Geometry: final body of the model. Coordinates: model frame, mm. A direction names the side the tool comes from. Round coordinates to 2 decimals unless told otherwise and drop trailing zeros. Order: outer loops, then holes, each group sorted by start corner. A loop starts at its lowest first (then second) coordinate and runs counter-clockwise, first axis right, second up. Notation, with made-up numbers: (-37, 17) -> (-27, 17) arc R20 cw to (-27, 25) -> close; hole circle Ø1 at (49.5, -30). An arc over 180 degrees is marked (long way). Put each result on its own line as item: value.
```python
from build123d import *

# Parameters (mm, degrees)
F0_R     = 3.048
F1_DEPTH = 3.175
F2_R     = 3.175


with BuildPart() as f1:
    # F0 (on Front) → F1 (new body)
    with BuildSketch(Plane.XZ):
        with BuildLine():
            ThreePointArc((-63.5, 3.175), (-62.570064, 0.929936), (-60.325, 0))
            Line((-60.325, 0), (60.325, 0))
            ThreePointArc((60.325, 0), (62.570064, 0.929936), (63.5, 3.175))
            Line((63.5, 3.175), (63.5, 27.559))
            ThreePointArc((63.5, 27.559), (62.570064, 29.804064), (60.325, 30.734))
            Line((60.325, 30.734), (7.62, 30.734))
            Line((7.62, 30.734), (-11.43, 26.924))
            Line((-11.43, 26.924), (-60.325, 26.924))
            ThreePointArc((-60.325, 26.924), (-62.570064, 25.994064), (-63.5, 23.749))
            Line((-63.5, 23.749), (-63.5, 3.175))
        make_face()
        with Locations((-40.64, 7.62)):
            Circle(F0_R, mode=Mode.SUBTRACT)
        with Locations((0, 7.62)):
            Circle(F0_R, mode=Mode.SUBTRACT)
        with Locations((40.64, 7.62)):
            Circle(F0_R, mode=Mode.SUBTRACT)
        with Locations((-53.34, 16.51)):
            Circle(F0_R, mode=Mode.SUBTRACT)
        with Locations((-25.4, 19.05)):
            Circle(F0_R, mode=Mode.SUBTRACT)
        with Locations((0, 19.05)):
            Circle(F0_R, mode=Mode.SUBTRACT)
        with Locations((25.4, 19.05)):
            Circle(F0_R, mode=Mode.SUBTRACT)
        with Locations((53.34, 16.51)):
            Circle(F0_R, mode=Mode.SUBTRACT)
    extrude(amount=F1_DEPTH)

    # F2
    f2_edges = [f1.edges().sort_by_distance(p)[0] for p in [
        (-11.43, -1.5875, 26.924),
        (7.62, -1.5875, 30.734),
    ]]
    fillet(f2_edges, radius=F2_R)


solid = f1.part
```
1. Cut plane C-C on y = -0.55. State how many separate pieces and enclosed holes the cut face has, and give its area (3 significant figures).
Ans:
separate pieces: 1
enclosed holes: 8
area: 3,430 mm²
2. Contact query for flat-ended pins moving along their axis: P1, Ø1.5, axis at x = -10.5, y = -1, coming from the +Z side; P2, Ø1, axis at y = -2, z = 26.5, coming from the -X side. Output: stop coordinate, or through.
Ans:
P1: z = 27.26
P2: x = -62.56
3. Cut plane D-D on x = 0. Return loops of the section in (y, z) (3 decimals).
Ans:
outline: (-3.175, 0) -> (0, 0) -> (0, 4.572) -> (-3.175, 4.572) -> close; (-3.175, 10.668) -> (0, 10.668) -> (0, 16.002) -> (-3.175, 16.002) -> close; (-3.175, 22.098) -> (0, 22.098) -> (0, 29.21) -> (-3.175, 29.21) -> close
4. Material intervals for probe 1 along Z at (x, y) = (25.4, -1.3); probe 2 along Z at (x, y) = (-25.4, -2.1); probe 3 along X at (y, z) = (-1.3, 21), sorted ascending.
Ans:
probe 1: 0 to 16, 22.1 to 30.73
probe 2: 0 to 16, 22.1 to 26.92
probe 3: -63.5 to -27.74, -23.06 to -2.34, 2.34 to 23.06, 27.74 to 63.5
5. Cut plane B-B on z = 7.62. Return loops of the section in (x, y) (3 decimals), and give its area (3 significant figures).
Ans:
outline: (-63.5, -3.175) -> (-43.688, -3.175) -> (-43.688, 0) -> (-63.5, 0) -> close; (-37.592, -3.175) -> (-3.048, -3.175) -> (-3.048, 0) -> (-37.592, 0) -> close; (3.048, -3.175) -> (37.592, -3.175) -> (37.592, 0) -> (3.048, 0) -> close; (43.688, -3.175) -> (63.5, -3.175) -> (63.5, 0) -> (43.688, 0) -> close
area: 345 mm²
6. Draft query along X for faces 3 (the face through (63.5, -2, 15)), 4 (the face through (-1.776, -1.565, 28.855)), 5 (the face through (-0.4, -1.57, 10.64)). Return one class per face: +X half, -X half, draft (parallel to the pull), parting line (faces both ways), or undercut.
Ans:
face 3: +X half
face 4: -X half
face 5: undercut
7. Cut plane A-A on x = -25.4. Return loops of the section in (y, z) (3 decimals), and give its area (3 significant figures).
Ans:
outline: (-3.175, 0) -> (0, 0) -> (0, 16.002) -> (-3.175, 16.002) -> close; (-3.175, 22.098) -> (0, 22.098) -> (0, 26.924) -> (-3.175, 26.924) -> close
area: 66.1 mm²
8. Set-up query: faces 1 (the face through (-36, -2, 26.924)), 2 (the face through (-1, -2, 0)). Return all of +Z, -Z, +X, -X, +Y, -Y with unobstructed straight access to the full face (end or side cutting, diameter ignored); none if empty.
Ans:
face 1: +Z, -X, +Y, -Y
face 2: -Z, +X, -X, +Y, -Y
